from build123d import *

# Parameters (mm, degrees)
BOSS_EXTRUDE1_DEPTH = 3.175
SKETCH3_R           = 2.4892
CUT_EXTRUDE1_DEPTH  = 4.175
SKETCH4_R           = 2.413
CUT_EXTRUDE2_DEPTH  = 4.175
SKETCH5_W           = 25.4
SKETCH5_H           = 12.7
CUT_EXTRUDE3_DEPTH  = 4.175


with BuildPart() as part:
    # Sketch2 → Boss-Extrude1 (new body)
    with BuildSketch(Plane.XY):
        Polygon((0, 0), (0, 63.5), (25.4, 63.5), (25.4, 25.4), (63.5, 25.4), (63.5, 0), align=None)
    extrude(amount=BOSS_EXTRUDE1_DEPTH)

    # Sketch3 → Cut-Extrude1 (cut, through all)
    with BuildSketch(Plane.XY.offset(3.175)):
        with Locations((16.419743879, 16.419743879)):
            Circle(SKETCH3_R)
        with Locations((12.7, 54.61)):
            Circle(SKETCH3_R)
        with Locations((12.7, 44.45)):
            Circle(SKETCH3_R)
        with Locations((34.29, 12.7)):
            Circle(SKETCH3_R)
        with Locations((54.61, 12.7)):
            Circle(SKETCH3_R)
        Polygon((0, 0), (0, 19.05), (19.05, 0), align=None)
    extrude(amount=-CUT_EXTRUDE1_DEPTH, mode=Mode.SUBTRACT)

    # Sketch4 → Cut-Extrude2 (cut, through all)
    with BuildSketch(Plane(origin=(0, 0, 0), x_dir=(-1, 0, 0), z_dir=(0, 0, -1))):
        with Locations((-12.7, 25.4)):
            Circle(SKETCH4_R)
    extrude(amount=-CUT_EXTRUDE2_DEPTH, mode=Mode.SUBTRACT)

    # Sketch5 → Cut-Extrude3 (cut, through all)
    with BuildSketch(Plane.XY.offset(3.175)):
        with Locations((12.7, 57.15)):
            Rectangle(SKETCH5_W, SKETCH5_H)
    extrude(amount=-CUT_EXTRUDE3_DEPTH, mode=Mode.SUBTRACT)


solid = part.part
The listing builds one solid part. Answer for the finished solid, in the listing's coordinates (mm). A direction names the side the tool comes from. Give positions to 0.01 mm unless a question says otherwise; leave off trailing zeros. Write each loop counter-clockwise with the first axis right and the second up, starting at its lowest first coordinate (ties: lowest second). Pieces come first, ordered by that corner, then holes. Notation, with made-up numbers: (10, -24.75) - (18, -24.75) arc R15 cw to (18, -2.75) - close; hole circle Ø3 at (38.5, 71). An arc over 180 degrees is marked (long way). One line per question, with ' | ' between items. Start each with the question number.
1. Section D-D, the plane z = 1.8 is taken. Determine the outline of the cut face in (x, y).
2. Given P1, Ø4.5, axis at x = 16.42, y = 16.42, coming from the -Z side; P2, Ø1, axis at x = 46, z = 1, coming from the +Y side; P3, Ø1.6, axis at y = 34, z = 1.5, coming from the +X side; P4, Ø1, axis at y = 13, z = 1.5, coming from the -X side, each flat-ended and moving along its own axis, determine where each tip first touches the part or whether it passes through.
3. Determine the mould class of faces 1 (the face through (11.587, 23.259, 1.565)), 2 (the face through (25.4, 38, 2)), 3 (the face through (42, 0, 2)) for opening direction Y: +Y half, -Y half, draft (parallel to the pull), parting line (faces both ways), or undercut.
4. Section B-B, the plane x = 54.61 is taken. Determine the outline of the cut face in (y, z) (3 decimals), then the cut area to 3 significant figures.
5. Section A-A, the plane x = 12.7 is taken. Determine the outline of the cut face in (y, z) (3 decimals).
6. Straight lines are drawn through the part: line 1 (Y direction, x = 54.61, z = 2.2); line 2 (Y direction, x = 12.7, z = 1.45); line 3 (Y direction, x = 11, z = 2.6). For each, find the intervals that lie inside material, in ascending order.
7. For faces 4 (the face through (25, 20, 3.175)), 5 (the face through (44, 25.4, 2)), determine the directions among +Z, -Z, +X, -X, +Y, -Y from which every point of the face is accessible in a straight line to the end or side of a thin tool.
Result:
1) outline: (0, 19.05) - (19.05, 0) - (63.5, 0) - (63.5, 25.4) - (25.4, 25.4) - (25.4, 50.8) - (0, 50.8) - close; hole circle Ø4.98 at (12.7, 44.45); hole circle Ø4.83 at (12.7, 25.4); hole circle Ø4.98 at (16.42, 16.42); hole circle Ø4.98 at (34.29, 12.7); hole circle Ø4.98 at (54.61, 12.7)
2) P1: passes through | P2: stops at y = 25.4 | P3: stops at x = 25.4 | P4: stops at x = 5.55
3) face 1: undercut | face 2: draft | face 3: -Y half
4) outline: (0, 0) - (10.211, 0) - (10.211, 3.175) - (0, 3.175) - close; (15.189, 0) - (25.4, 0) - (25.4, 3.175) - (15.189, 3.175) - close | area: 64.8 mm2
5) outline: (6.35, 0) - (22.987, 0) - (22.987, 3.175) - (6.35, 3.175) - close; (27.813, 0) - (41.961, 0) - (41.961, 3.175) - (27.813, 3.175) - close; (46.939, 0) - (50.8, 0) - (50.8, 3.175) - (46.939, 3.175) - close
6) line 1: y = 0 to 10.21, 15.19 to 25.4 | line 2: y = 6.35 to 22.99, 27.81 to 41.96, 46.94 to 50.8 | line 3: y = 8.05 to 23.69, 27.11 to 42.63, 46.27 to 50.8
7) face 4: +Z, +X, -X, +Y, -Y | face 5: +Z, -Z, +X, +Y
